Answer from the drawing. Dimensions are ordinates in mm from the lowest x, y and z of the part. A direction names the side the tool comes from. Round coordinates to 2 decimals unless told otherwise and drop trailing zeros. Write each loop counter-clockwise with the first axis right and the second up, starting at its lowest first coordinate (ties: lowest second). Pieces come first, ordered by that corner, then holes. Notation, with made-up numbers: (72.25, 8) -> (109.25, 8) arc R14 cw to (109.25, 16) -> close; hole circle Ø3 at (-32, 61). An arc over 180 degrees is marked (long way). Return JSON: item names as keys, results as strings. Group by question number.
(1) Given pin 1 (3 mm diameter, centred on x = 9, z = 8, fed in from -Y); pin 2 (1.3 mm diameter, centred on y = 1.5, z = 6.5, fed in from +X); pin 3 (2 mm diameter, centred on y = 14.5, z = 7.5, fed in from +X), each flat-ended and moving along its own axis, determine where each tip first touches the part or whether it passes through.
(2) A cutting plane is placed at C-C on x = 8.25. Give the vertices of the cut face in (y, z), then the cut area to 3 significant figures.
(3) A cutting plane is placed at B-B on z = 3. Give the vertices of the cut face in (x, y).
(4) For the marked faces 4, 5 and 6, determine the directions among +Z, -Z, +X, -X, +Y, -Y from which every point of the face is accessible in a straight line to the end or side of a thin tool.
(5) The mould has two halves that part along Z. Classify the marked faces 1, 2 and 3: released by +Z, released by -Z, zero draft, split by the parting line, or undercut.
(6) Straight lines are drawn through the part: line 1 (Y direction, x = 2.75, z = 6.35); line 2 (Y direction, x = 12.25, z = 6); line 3 (X direction, y = 12, z = 0.5). For each, find the intervals that lie inside material, in ascending order.
(7) A cutting plane is placed at A-A on z = 6.35. Give the vertices of the cut face in (x, y).
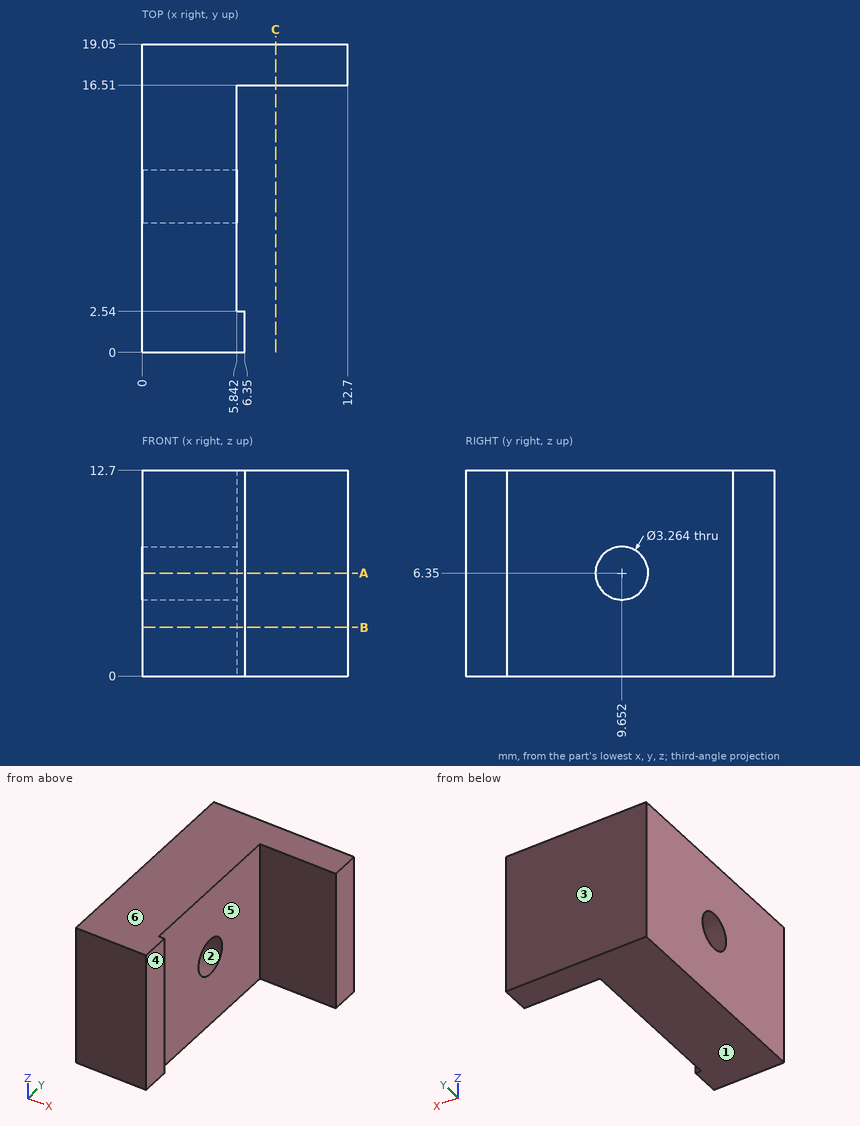
Checks:
{
 "1": {"pin 1": "stops at y = 16.51", "pin 2": "stops at x = 6.35", "pin 3": "stops at x = 5.84"},
 "2": {"outline": "(16.51, 0) -> (19.05, 0) -> (19.05, 12.7) -> (16.51, 12.7) -> close", "area": "32.3 mm^2"},
 "3": {"outline": "(0, 0) -> (6.35, 0) -> (6.35, 2.54) -> (5.84, 2.54) -> (5.84, 16.51) -> (12.7, 16.51) -> (12.7, 19.05) -> (0, 19.05) -> close"},
 "4": {"face 4": "+Z, -Z, +X, -Y", "face 5": "+Z, -Z, +X", "face 6": "+Z, +X, -X, +Y, -Y"},
 "5": {"face 1": "released by -Z", "face 2": "undercut", "face 3": "zero draft"},
 "6": {"line 1": "y = 0 to 8.02, 11.28 to 19.05", "line 2": "y = 16.51 to 19.05", "line 3": "x = 0 to 5.84"},
 "7": {"outline": "(0, 0) -> (6.35, 0) -> (6.35, 2.54) -> (5.84, 2.54) -> (5.84, 8.02) -> (0, 8.02) -> close; (0, 11.28) -> (5.84, 11.28) -> (5.84, 16.51) -> (12.7, 16.51) -> (12.7, 19.05) -> (0, 19.05) -> close"}
}
